Can you work these out from the model? Positions are in its coordinate system, mm. Face numbers are marked on the shaded views. A direction names the side the tool comes from. Coordinates: 2 decimals unless noted, no trailing zeros. Order: outer loops, then holes, each group sorted by start corner. A loop starts at its lowest first (then second) coordinate and runs counter-clockwise, first axis right, second up. Notation, with made-up numbers: (58.25, 17.5) - (111.25, 17.5) arc R22 cw to (111.25, 44.5) - close; hole circle Ø6 at (79, -23). An arc over 180 degrees is marked (long way). Use a Markdown table: item, result. Add a question column.
(1) I want a section at D-D (x = 7). List the corners of the cut face in (y, z) for me, and give its area (3 significant figures).
(2) I want a section at A-A (z = 0). List the corners of the cut face in (x, y) for me.
(3) I want a section at B-B (x = -621.47). List the corners of the cut face in (y, z) for me.
(4) For pin 1 Ø12 at (y, z) = (85.5, 16) entering from +X; pin 2 Ø5 at (x, z) = (-446, 43) entering from +Y, each with a flat end and sliding along its axis, tell me the tip position at first contact or that it passes through.
(5) If I drill on L1, parallel to Y at x = -115, z = 63, over which ranges is the centre line in solid material (lowest first)? Write a range as [from, to].
(6) I want a section at C-C (y = 83). List the corners of the cut face in (x, z) for me, and give its area (3 significant figures).
(7) We'd pull the mould along X, two halves only. Please class the marked faces 3, 4 and 5: pulls with the +X half, pulls with the -X half, needs draft (parallel to the pull), parting line crosses it, or undercut.
(8) On a 3-axis mill with a long thin cutter (end or side, diameter ignored), from which of +Z, -Z, +X, -X, +Y, -Y can I reach the whole of each face in a straight line? I mean the marked faces 1 and 2. Say none if no direction works.
```python
from build123d import *

# Parameters (mm, degrees)
BOSS_EXTRUDE1_DEPTH = 50.8
SKETCH2_R           = 29.86
BOSS_EXTRUDE2_DEPTH = 152.4


with BuildPart() as part:
    # Sketch1 → Boss-Extrude1 (new body)
    with BuildSketch(Plane(origin=(0, 0, 0), x_dir=(1, 0, 0), z_dir=(0, 1, 0))):
        with BuildLine():
            Line((67.96, 0), (29.86, 0))
            ThreePointArc((29.86, 0), (0, -29.86), (-29.86, 0))
            Line((-29.86, 0), (-591.61, 0))
            ThreePointArc((-591.61, 0), (-621.47, -29.86), (-651.33, 0))
            Line((-651.33, 0), (-689.43, 0))
            Line((-689.43, 0), (-689.43, -76.2))
            Line((-689.43, -76.2), (67.96, -76.2))
            Line((67.96, -76.2), (67.96, 0))
        make_face()
        with BuildLine():
            ThreePointArc((-29.86, 0), (0, 29.86), (29.86, 0))
            Line((29.86, 0), (67.96, 0))
            Line((67.96, 0), (67.96, 76.2))
            Line((67.96, 76.2), (-689.43, 76.2))
            Line((-689.43, 76.2), (-689.43, 0))
            Line((-689.43, 0), (-651.33, 0))
            ThreePointArc((-651.33, 0), (-621.47, 29.86), (-591.61, 0))
            Line((-591.61, 0), (-29.86, 0))
        make_face()
    extrude(amount=BOSS_EXTRUDE1_DEPTH)

    # Sketch2 → Boss-Extrude2 (add)
    with BuildSketch(Plane.XZ):
        with Locations(Location((0, 0, 0), (0, 0, 270))):
            Circle(SKETCH2_R)
        with Locations(Location((-621.47, 0, 0), (0, 0, 270))):
            Circle(SKETCH2_R)
    extrude(amount=-BOSS_EXTRUDE2_DEPTH)


solid = part.part
```
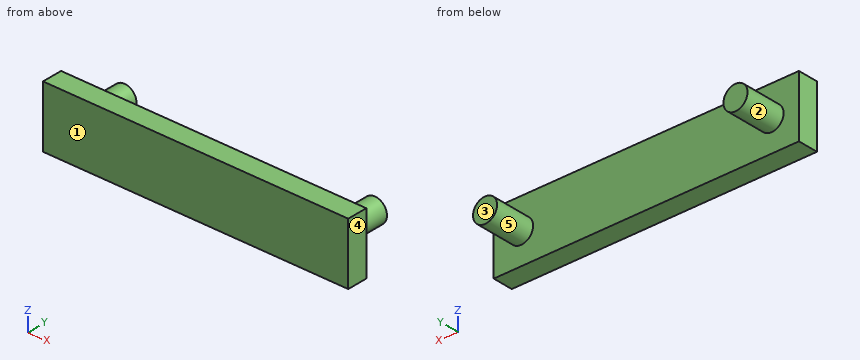
Answers follow:
| question | item | result |
|---|---|---|
| 1 | outline | (0, -76.2) - (50.8, -76.2) - (50.8, -29.03) - (152.4, -29.03) - (152.4, 29.03) - (50.8, 29.03) - (50.8, 76.2) - (0, 76.2) - close |
| 1 | area | 13,600 mm² |
| 2 | outline | (-689.43, 0) - (67.96, 0) - (67.96, 50.8) - (29.86, 50.8) - (29.86, 152.4) - (-29.86, 152.4) - (-29.86, 50.8) - (-591.61, 50.8) - (-591.61, 152.4) - (-651.33, 152.4) - (-651.33, 50.8) - (-689.43, 50.8) - close |
| 3 | outline | (0, -76.2) - (50.8, -76.2) - (50.8, -29.86) - (152.4, -29.86) - (152.4, 29.86) - (50.8, 29.86) - (50.8, 76.2) - (0, 76.2) - close |
| 4 | pin 1 | stops at x = 28.14 |
| 4 | pin 2 | stops at y = 50.8 |
| 5 | L1 | y = [0, 50.8] |
| 6 | outline | circle Ø59.72 at (-621.47, 0); circle Ø59.72 at (0, 0) |
| 6 | area | 5,600 mm² |
| 7 | face 3 | needs draft |
| 7 | face 4 | pulls with the +X half |
| 7 | face 5 | undercut |
| 8 | face 1 | +Z, -Z, +X, -X, -Y |
| 8 | face 2 | +Y |
